from build123d import *

# Parameters (mm, degrees)
SKETCH_1_R          = 12.25
SKETCH_1_R_2        = 1.25
EXTRUDE_1_DEPTH     = 2
SKETCH_2_R          = 3
EXTRUDE_2_DEPTH     = 10.63
SKETCH_3_W          = 2
SKETCH_3_H          = 12
EXTRUDE_3_DEPTH     = 8
SKETCH_5_R          = 1.6
CUT_EXTRUDE_1_DEPTH = 10
SKETCH_6_W          = 6
SKETCH_6_H          = 12
EXTRUDE_4_DEPTH     = 10.63
SKETCH_7_W          = 4
SKETCH_7_H          = 12
CUT_EXTRUDE_2_DEPTH = 2
SKETCH_8_R          = 12.25
CUT_EXTRUDE_3_DEPTH = 8
SKETCH_9_R          = 3
EXTRUDE_5_DEPTH     = 25


with BuildPart() as part:
    # 草图1 → 凸台-拉伸1 (new body)
    with BuildSketch(Plane(origin=(0, 0, 0), x_dir=(1, 0, 0), z_dir=(0, 1, 0))):
        Circle(SKETCH_1_R)
        with Locations((8, 0)):
            Circle(SKETCH_1_R_2, mode=Mode.SUBTRACT)
        with Locations((0, -8)):
            Circle(SKETCH_1_R_2, mode=Mode.SUBTRACT)
        with Locations((-8, 0)):
            Circle(SKETCH_1_R_2, mode=Mode.SUBTRACT)
        with Locations((0, 8)):
            Circle(SKETCH_1_R_2, mode=Mode.SUBTRACT)
    extrude(amount=EXTRUDE_1_DEPTH)

    # 草图2 → 凸台-拉伸2 (add)
    with BuildSketch(Plane(origin=(0, 2, 0), x_dir=(1, 0, 0), z_dir=(0, 1, 0))):
        Circle(SKETCH_2_R)
    extrude(amount=EXTRUDE_2_DEPTH)

    # 草图3 → 凸台-拉伸3 (add)
    with BuildSketch(Plane(origin=(0, 12.63, 0), x_dir=(1, 0, 0), z_dir=(0, 1, 0))):
        with Locations((-2, 0)):
            Rectangle(SKETCH_3_W, SKETCH_3_H)
    extrude(amount=EXTRUDE_3_DEPTH)

    # 草图5 → 切除-拉伸1 (cut)
    with BuildSketch(Plane(origin=(-1, 0, 0), x_dir=(0, 0, -1), z_dir=(1, 0, 0))):
        with Locations((3, 16.63)):
            Circle(SKETCH_5_R)
        with Locations((-3, 16.63)):
            Circle(SKETCH_5_R)
    extrude(amount=-CUT_EXTRUDE_1_DEPTH, mode=Mode.SUBTRACT)

    # 草图6 → 凸台-拉伸4 (add)
    with BuildSketch(Plane(origin=(0, 2, 0), x_dir=(1, 0, 0), z_dir=(0, 1, 0))):
        Rectangle(SKETCH_6_W, SKETCH_6_H)
    extrude(amount=EXTRUDE_4_DEPTH)

    # 草图7 → 切除-拉伸2 (cut)
    with BuildSketch(Plane(origin=(0, 12.63, 0), x_dir=(1, 0, 0), z_dir=(0, 1, 0))):
        with Locations((1, 0)):
            Rectangle(SKETCH_7_W, SKETCH_7_H)
    extrude(amount=-CUT_EXTRUDE_2_DEPTH, mode=Mode.SUBTRACT)

    # 草图8 → 切除-拉伸3 (cut)
    with BuildSketch(Plane.XZ):
        Circle(SKETCH_8_R)
    extrude(amount=-CUT_EXTRUDE_3_DEPTH, mode=Mode.SUBTRACT)

    # 草图9 → 凸台-拉伸5 (add)
    with BuildSketch(Plane.XZ.offset(-8)):
        Circle(SKETCH_9_R)
    extrude(amount=EXTRUDE_5_DEPTH)


solid = part.part
CAD build for the part. Positions are in the model's coordinates, mm. A direction names the side the tool comes from. Coordinates: 2 decimals unless noted, no trailing zeros. Write each loop counter-clockwise with the first axis right and the second up, starting at its lowest first coordinate (ties: lowest second). Pieces come first, ordered by that corner, then holes. Notation, with made-up numbers: M 69.5,78 L 109.5,78 A18 ccw 109.5,105 Z; hole C 47,2.25 d6. An arc over 180 degrees is marked long. Answer as a JSON object with one key per item and string values. Group by question number.
1) Saw through at A-A (z = -2). Write the cut outline in (x, y).
2) Pin check, flat tips, straight feed: pin 1 Ø4 at (y, z) = (16.63, 3) entering from +X; pin 2 Ø2 at (x, z) = (0.5, 2) entering from +Y; pin 3 Ø4 at (y, z) = (3.5, 3.5) entering from -X. Stop position of each tip, or through.
3) Saw through at D-D (x = -1.85). Write the cut outline in (y, z).
4) Wall check: line 1 (Y direction, x = -1.8, z = -3); line 2 (X direction, y = 14, z = -2); line 3 (Z direction, x = 0.1, y = -13). Give the ranges that are in metal, low to high. Write a range as from..to.
5) Saw through at B-B (y = 16.63). Write the cut outline in (x, z).
6) Tool access for faces 4 (the face through (-3, -4, 0)), 5 (the face through (0, 8, -4)), 6 (the face through (1, 10.63, 0)): list every direction of +Z, -Z, +X, -X, +Y, -Y with a clear straight run to the whole face (end or side of a thin tool).
7) Saw through at C-C (x = 1). Write the cut outline in (y, z), plus the area to 3 significant figures.
8) Mould opens along Y. For faces 1 (the face through (-1.986, 18.216, -2.792)), 2 (the face through (-1.4, 12.8, 6)), 3 (the face through (0, 8, 4)) say: +Y half, -Y half, draft (parallel to the pull), parting line (faces both ways), or undercut.
Values follow:
{
 "1": {"outline": "M -3,8 L -2.24,8 L -2.24,-17 L 2.24,-17 L 2.24,8 L 3,8 L 3,10.63 L -1,10.63 L -1,15.38 L -3,15.38 Z; M -3,17.88 L -1,17.88 L -1,20.63 L -3,20.63 Z"},
 "2": {"pin 1": "stops at x = -1", "pin 2": "stops at y = 10.63", "pin 3": "stops at x = -2.6"},
 "3": {"outline": "M -17,-2.36 L 8,-2.36 L 8,-6 L 20.63,-6 L 20.63,6 L 8,6 L 8,2.36 L -17,2.36 Z; hole C 16.63,-3 d3.2; hole C 16.63,3 d3.2"},
 "4": {"line 1": "y = 8..15.03, 18.23..20.63", "line 2": "x = -3..-1", "line 3": "z = -3..3"},
 "5": {"outline": "M -3,-6 L -1,-6 L -1,-4.6 L -3,-4.6 Z; M -3,-1.4 L -1,-1.4 L -1,1.4 L -3,1.4 Z; M -3,4.6 L -1,4.6 L -1,6 L -3,6 Z"},
 "6": {"face 4": "-Y", "face 5": "-Z, -Y", "face 6": "+Z, -Z, +X, +Y"},
 "7": {"outline": "M -17,-2.83 L 8,-2.83 L 8,-6 L 10.63,-6 L 10.63,6 L 8,6 L 8,2.83 L -17,2.83 Z", "area": "173 mm2"},
 "8": {"face 1": "undercut", "face 2": "draft", "face 3": "-Y half"}
}
